Model file for the job. Use its own axes, mm. Round coordinates to 2 decimals unless told otherwise and drop trailing zeros. Order: outer loops, then holes, each group sorted by start corner. A loop starts at its lowest first (then second) coordinate and runs counter-clockwise, first axis right, second up. Notation, with made-up numbers: M 10.25,49 L 54.25,49 A3 ccw 54.25,53 Z; hole C -16,49.5 d5. An arc over 180 degrees is marked long. Return JSON: item names as keys, results as strings. Group by question number.
Item 1: Probe line 1 along X through (y, z) = (9, -76.2); line 2 along Z through (x, y) = (-188.5, 6.5); line 3 along Z through (x, y) = (-217, 6.75). List the from-to ranges inside material, lowest first.
Item 2: Slice it at C-C on y = 8. Give the number of separate pieces and of enclosed holes in the cut face, then the cut area to 3 significant figures.
Item 3: Slice it at B-B on x = -177. Write the cut outline in (y, z).
Item 4: Slice it at A-A on z = -76.2. Write the cut outline in (x, y), then the cut area to 3 significant figures.
Autodesk Inventor part; units mm, degrees
ref_plane "YZ Plane" through (0, 0, 0) normal (1, 0, 0) x (0, 1, 0)
ref_plane "XZ Plane" through (0, 0, 0) normal (0, 1, 0) x (-1, 0, 0)
ref_plane "XY Plane" through (0, 0, 0) normal (0, 0, 1) x (1, 0, 0)
sketch "Sketch1" plane through (0, 0, 0) normal (0, 1, 0) x (-1, 0, 0)
  line L0 (0, 0) -> (253.2063, 0)
  line L1 (253.2063, 0) -> (253.2063, -152.4)
  line L2 (253.2063, -152.4) -> (0, -152.4)
  line L3 (0, -152.4) -> (0, 0)
  line L4 (0, -76.2) -> (56.3563, -76.2)
  circle A0 centre (56.3563, -76.2) radius 4.7625
  dimension "d0" = 152.4
  dimension "d1" = 253.2063
  dimension "d2" = 56.3563
  dimension "d3" = 9.525
extrude "Extrusion1" add sketch "Sketch1" along normal blind 11.9062
sketch "Sketch2" plane through (0, 11.9062, 0) normal (0, 1, 0) x (1, 0, 0)
  line L0 (0, 0) -> (0, 152.4)
  line L1 (0, 76.2) -> (-177.0063, 76.2)
  circle A0 centre (-177.0063, 76.2) radius 6.35
  line L2 (-177.0063, 76.2) -> (-215.1063, 76.2)
  circle A1 centre (-215.1063, 76.2) radius 6.35
  circle A2 centre (-188.7798, 39.9647) radius 6.35
  circle A3 centre (-146.1827, 53.8054) radius 6.35
  circle A4 centre (-146.1827, 98.5946) radius 6.35
  circle A5 centre (-188.7798, 112.4353) radius 6.35
  dimension "d6" = 12.7
  dimension "d7" = 38.1
  dimension "d8" = 12.7
  dimension "d11" = 360
  dimension "d13" = 177.0062
extrude "Extrusion2" cut sketch "Sketch2" against normal blind 11.9062
properties part number "Stage3Wall" material "Wood (Birch)"
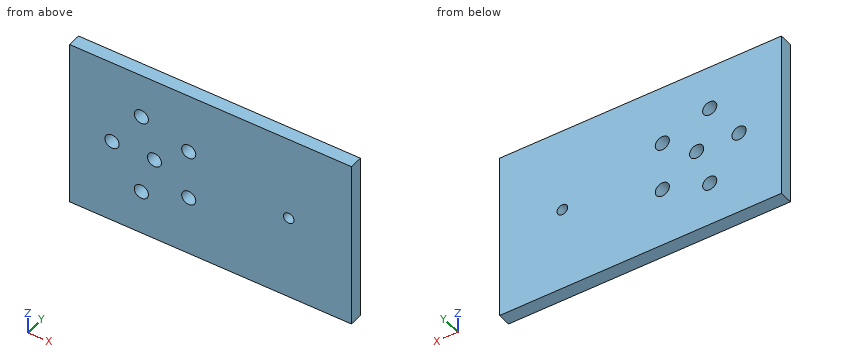
Output values:
{
 "1": {"line 1": "-253.21 to -221.46, -208.76 to -183.36, -170.66 to -61.12, -51.59 to 0", "line 2": "-152.4 to -118.78, -106.09 to -46.31, -33.62 to 0", "line 3": "-152.4 to -82.26, -70.14 to 0"},
 "2": {"separate pieces": "1", "enclosed holes": "7", "area": "37,800 mm²"},
 "3": {"outline": "M 0,-152.4 L 11.91,-152.4 L 11.91,-82.55 L 0,-82.55 Z; M 0,-69.85 L 11.91,-69.85 L 11.91,0 L 0,0 Z"},
 "4": {"outline": "M -253.21,0 L -221.46,0 L -221.46,11.91 L -253.21,11.91 Z; M -208.76,0 L -183.36,0 L -183.36,11.91 L -208.76,11.91 Z; M -170.66,0 L -61.12,0 L -61.12,11.91 L -170.66,11.91 Z; M -51.59,0 L 0,0 L 0,11.91 L -51.59,11.91 Z", "area": "2,600 mm²"}
}
